Check sheet for the modelled part. Datum: model origin and axes. Units: mm. A direction names the side the tool comes from. Give positions to 0.01 mm unless a question says otherwise; leave off trailing zeros. Write each loop counter-clockwise with the first axis right and the second up, starting at its lowest first coordinate (ties: lowest second). Pieces come first, ordered by that corner, then holes. Notation, with made-up numbers: M 29,16 L 73,16 A14 cw 73,25 Z; hole C 72,-9.75 d1. An arc over 180 degrees is marked long. Write item = value, one per line. Start each with the question number.
1) Sectioned sample at C-C, the plane y = -69. Record the cut outline in (x, z), then the cut area to 3 significant figures.
2) Sectioned sample at A-A, the plane z = 38.5. Record the cut outline in (x, y), then the cut area to 3 significant figures.
3) Draft check along Z on faces 1 (the face through (40.336, -26.928, 81.674)), 2 (the face through (28, -52, 101.6)), 3 (the face through (54, -50, 31.984)). Enter one of: pulls with the +Z half, pulls with the -Z half, needs draft (parallel to the pull), parting line crosses it, or undercut.
4) Sectioned sample at D-D, the plane x = 66. Record the cut outline in (y, z), then the cut area to 3 significant figures.
5) Sectioned sample at B-B, the plane x = 84.5. Record the cut outline in (y, z).
6) Set-up check for faces 4 (the face through (87.211, -50, 47)), 5 (the face through (0, -52, 50)), 6 (the face through (66.474, -74.751, 82.225)): record each of +Z, -Z, +X, -X, +Y, -Y from which the full face is reachable in a straight line by a thin tool's end or side.
7) Scan lines: L1, parallel to Y at x = 60, z = 84.5; L2, parallel to Z at x = 37, y = -42.5; L3, parallel to X at y = -33.5, z = 73.5. Record each from-to range of solid material in increasing order.
from build123d import *

# Parameters (mm, degrees)
F0_W     = 101.6
F0_H     = 101.6
F1_DEPTH = 50.8
F2_W     = 17.7085362375
F2_H     = 30.314616859
F2_W_2   = 19.2092582583
F3_DEPTH = 25.4
F5_R     = 5.08


with BuildPart() as f1:
    # F0 (on Front) → F1 (new body)
    with BuildSketch(Plane.XZ):
        with Locations((50.8, 50.8)):
            Rectangle(F0_W, F0_H)
    extrude(amount=F1_DEPTH)

    # F2 (on face) → F3 (cut)
    with BuildSketch(Plane.XZ.offset(50.8)):
        Polygon((68.001665175, 101.6), (38.8876236975, 101.6), (38.8876236975, 62.298912555), (38.8876236975, 31.984295696), (68.001665175, 31.984295696), (68.001665175, 62.298912555), align=None)
        with Locations((30.0333555788, 47.1416041255)):
            Rectangle(F2_W, F2_H)
        with Locations((77.6062943041, 47.1416041255)):
            Rectangle(F2_W_2, F2_H)
    extrude(amount=-F3_DEPTH, mode=Mode.SUBTRACT)

    # F4: F1 across face


with BuildPart() as f1_1:
    add(f1.part)
    add(f1.part.mirror(Plane(origin=(49.4313994673, -50.8, 46.8540587323), x_dir=(1, 0, 0), z_dir=(0, -1, 0))))

    # F5
    f5_edges = [f1_1.edges().sort_by_distance(p)[0] for p in [
        (68.001665, -25.4, 81.949456),
        (38.887624, -25.4, 81.949456),
        (68.001665, -76.2, 81.949456),
        (38.887624, -76.2, 81.949456),
    ]]
    fillet(f5_edges, radius=F5_R)


solid = f1_1.part
Data:
q1.outline = M 0,0 L 101.6,0 L 101.6,101.6 L 68,101.6 L 68,62.3 L 87.21,62.3 L 87.21,31.98 L 21.18,31.98 L 21.18,62.3 L 38.89,62.3 L 38.89,101.6 L 0,101.6 Z
q1.area = 7,180 mm2
q2.outline = M 0,-101.6 L 101.6,-101.6 L 101.6,0 L 0,0 Z; hole M 21.18,-76.2 L 87.21,-76.2 L 87.21,-25.4 L 21.18,-25.4 Z
q2.area = 6,970 mm2
q3.face_1 = needs draft
q3.face_2 = pulls with the +Z half
q3.face_3 = undercut
q4.outline = M -101.6,0 L 0,0 L 0,101.6 L -26.44,101.6 L -26.44,62.3 L -25.4,62.3 L -25.4,31.98 L -76.2,31.98 L -76.2,62.3 L -75.16,62.3 L -75.16,101.6 L -101.6,101.6 Z
q4.area = 6,870 mm2
q5.outline = M -101.6,0 L 0,0 L 0,101.6 L -101.6,101.6 Z; hole M -76.2,31.98 L -25.4,31.98 L -25.4,62.3 L -76.2,62.3 Z
q6.face_4 = none
q6.face_5 = +Z, -Z, -X, +Y, -Y
q6.face_6 = +Z
q7.L1 = -101.6 to -76.2, -25.4 to 0
q7.L2 = 0 to 31.98, 62.3 to 101.6
q7.L3 = 0 to 38.89, 68 to 101.6
